```python
from build123d import *

# Parameters (mm, degrees)
F0_R     = 14.5796
F1_DEPTH = 4.826
F2_R     = 14.5796
F2_R_2   = 12.9286
F3_DEPTH = 1.524
F4_SIZE  = 0.762


with BuildPart() as f1:
    # F0 (on Top) → F1 (new body)
    with BuildSketch(Plane.XY):
        Circle(F0_R)
    extrude(amount=F1_DEPTH)

    # F2 (on face) → F3 (join)
    with BuildSketch(Plane.XY.offset(4.826)):
        Circle(F2_R)
        Circle(F2_R_2, mode=Mode.SUBTRACT)
    extrude(amount=F3_DEPTH)

    # F4
    f4_edges = [f1.edges().sort_by_distance(p)[0] for p in [
        (-12.9286, 0, 6.35),
    ]]
    chamfer(f4_edges, length=F4_SIZE)


solid = f1.part
```
The listing builds one solid part. Answer for the finished solid, in the listing's coordinates (mm). A direction names the side the tool comes from. Coordinates: 2 decimals unless noted, no trailing zeros. Write each loop counter-clockwise with the first axis right and the second up, starting at its lowest first coordinate (ties: lowest second). Pieces come first, ordered by that corner, then holes. Notation, with made-up numbers: (-11.75, 17.25) - (36.25, 17.25) arc R8 ccw to (36.25, 21.25) - close; hole circle Ø6 at (10.25, 61). An arc over 180 degrees is marked (long way). One line per item, written item: value.
1) Find section C-C (z = 2). Give the vertices of the cut face in (x, y), and give its area (3 significant figures).
Geometry check:
outline: circle Ø29.16 at (0, 0)
area: 668 mm2
2) For a pull along Y with two mould halves and no side action, classify faces 3 (the cylindrical face through (-1.68, 12.82, 5.2)), 4 (the cylindrical face through (-11.57, -8.87, 3.13)), 5 (the flat face through (0, 0, 0)) as pulls with the +Y half, pulls with the -Y half, needs draft (parallel to the pull), parting line crosses it, or undercut.
Geometry check:
face 3: undercut
face 4: parting line crosses it
face 5: needs draft
3) Consider line 1 along Y through (x, z) = (0, 5.05); line 2 along Y through (x, z) = (1.5, 6); line 3 along Z through (x, y) = (4.5, -3.5). Determine where each line is inside the solid, lowest interval first. Write a range as from..to.
Geometry check:
line 1: y = -14.58..-12.93, 12.93..14.58
line 2: y = -14.5..-13.26, 13.26..14.5
line 3: z = 0..4.83
4) Find section A-A (y = 0). Give the vertices of the cut face in (x, z).
Geometry check:
outline: (-14.58, 0) - (14.58, 0) - (14.58, 6.35) - (13.69, 6.35) - (12.93, 5.59) - (12.93, 4.83) - (-12.93, 4.83) - (-12.93, 5.59) - (-13.69, 6.35) - (-14.58, 6.35) - close
5) A tool of negligible diameter and unlimited length cuts with its end or side. For faces 1 (the flat face through (0, 0, 4.826)), 2 (the flat face through (9, -11, 6.35)), from which of +Z, -Z, +X, -X, +Y, -Y can it reach the whole face along a straight path? Write none if from no direction.
Geometry check:
face 1: +Z
face 2: +Z, +X, -X, +Y, -Y
6) Each of these flat-tipped pins is pushed along its axis until it touches: pin 1 Ø8 at (x, y) = (4, -5.5) entering from +Z; pin 2 Ø1 at (y, z) = (-6, 2) entering from +X; pin 3 Ø1 at (y, z) = (9, 5.5) entering from -X. Where does it stop, or does it pass through?
Geometry check:
pin 1: stops at z = 4.83
pin 2: stops at x = 13.5
pin 3: stops at x = -11.85
